```python
from build123d import *

# Parameters (mm, degrees)
SKETCH2_R          = 1
CUT_EXTRUDE1_DEPTH = 10.16


with BuildPart() as part:
    # Sketch1 → Revolve1 (revolve)
    with BuildSketch(Plane(origin=(0, 0, 0), x_dir=(0, 0, -1), z_dir=(1, 0, 0))):
        Polygon((0, 0), (-13.257279683, 0), (-13.85, 2.503549111), (-13.85, 13.261063329), (-11.086941731, 15.2), (-5, 15.2), (-5, 16.2), (-2.5, 16.2), (-2.5, 26.2), (0, 26.2), align=None)
    revolve(axis=Axis((0, 26.2, 0), (0, -1, 0)))

    # Sketch2 → Cut-Extrude1 (cut)
    with BuildSketch(Plane.XZ):
        with Locations(Location((0, 6, 0), (0, 0, 270))):
            Circle(SKETCH2_R)
        with Locations(Location((8, 0, 0), (0, 0, 270))):
            Circle(SKETCH2_R)
        with Locations(Location((0, -6, 0), (0, 0, 270))):
            Circle(SKETCH2_R)
        with Locations(Location((-8, 0, 0), (0, 0, 270))):
            Circle(SKETCH2_R)
    extrude(amount=-CUT_EXTRUDE1_DEPTH, mode=Mode.SUBTRACT)


solid = part.part
```
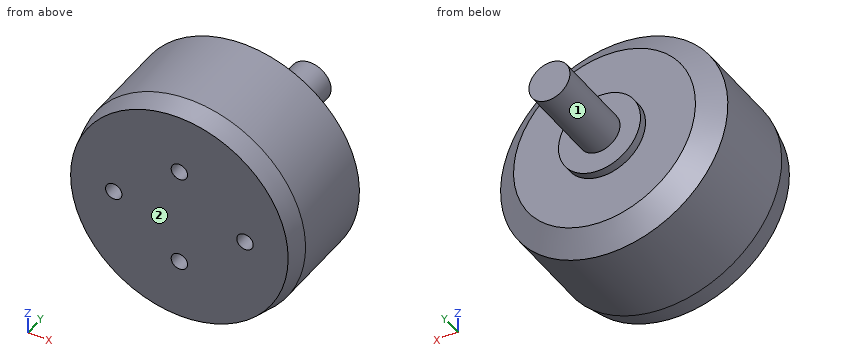
Input: part model. Units: mm. Frame: model coordinates. Face numbers are marked on the shaded views. A direction names the side the tool comes from. Coordinates: 2 decimals unless noted, no trailing zeros. Write each loop counter-clockwise with the first axis right and the second up, starting at its lowest first coordinate (ties: lowest second). Pieces come first, ordered by that corner, then holes. Notation, with made-up numbers: (79, -35) -> (125, -35) arc R26 cw to (125, 3) -> close; hole circle Ø1 at (-6, -9). An arc over 180 degrees is marked (long way). Answer as a JSON object with one key per item and string values.
1. First-contact query: P1, Ø1.8, axis at x = 0, z = 6, coming from the +Y side; P2, Ø0.6, axis at x = 0, z = 6, coming from the -Y side; P3, Ø2, axis at x = 2, y = 10.5, coming from the -Z side. Flat tips, straight axial feed; report the tip coordinate or a pass-through.
Result set:
{"P1": "stops at y = 15.2", "P2": "stops at y = 10.16", "P3": "stops at z = -13.81"}
2. Section B-B on y = 20. Return the cut outline in (x, z), then the cut area to 3 significant figures.
Result set:
{"outline": "circle Ø5 at (0, 0)", "area": "19.6 mm2"}
3. Material intervals for line 1 (X direction, y = 3.75, z = 0); line 2 (X direction, y = 1.75, z = 0.75); line 3 (Y direction, x = 5.5, z = -5.5), sorted ascending. Write a range as from..to.
Result set:
{"line 1": "x = -13.85..-9, -7..7, 9..13.85", "line 2": "x = -13.65..-8.66, -7.34..7.34, 8.66..13.65", "line 3": "y = 0..15.2"}
4. Section A-A on y = 5. Return the cut outline in (x, z).
Result set:
{"outline": "circle Ø27.7 at (0, 0); hole circle Ø2 at (-8, 0); hole circle Ø2 at (0, -6); hole circle Ø2 at (0, 6); hole circle Ø2 at (8, 0)"}
5. Access query for the marked faces 1 and 2. Directions: +Z, -Z, +X, -X, +Y, -Y. A direction counts if a zero-diameter tool reaches every point of the face in a straight line with its end or side. Return the directions, or none.
Result set:
{"face 1": "+Y", "face 2": "+Z, -Z, +X, -X, -Y"}
